The model under review builds one solid part; all positions refer to its coordinate system, in mm. Face numbers are marked on the shaded views. Coordinates: 2 decimals unless noted, no trailing zeros. Loops run counter-clockwise (first coordinate to the right, second up) from the corner with the lowest first, then second, coordinate; pieces in that order, holes last. Notation, with made-up numbers: M 65,-35 L 113,-35 A26 cw 113,-10 Z; hole C 10.5,32 d8. An arc over 180 degrees is marked long. Use CSV: the item, a comma, the result in double quotes. Start each with the question number.
from build123d import *

# Parameters (mm, degrees)
SKETCH1_R           = 4
SKETCH1_R_2         = 2.45
BOSS_EXTRUDE1_DEPTH = 8
SKETCH2_R           = 6
BOSS_EXTRUDE2_DEPTH = 2
FILLET1_R           = 1
CUT_EXTRUDE1_REACH  = 15.115
SKETCH3_R           = 2.45
CHAMFER1_SIZE       = 1


with BuildPart() as part:
    # Sketch1 → Boss-Extrude1 (new body)
    with BuildSketch(Plane(origin=(0, 0, 0), x_dir=(1, 0, 0), z_dir=(0, 1, 0))):
        with Locations(Location((0, 0, 0), (0, 0, 270))):
            Circle(SKETCH1_R)
        with Locations(Location((0, 0, 0), (0, 0, 270))):
            Circle(SKETCH1_R_2, mode=Mode.SUBTRACT)
    extrude(amount=BOSS_EXTRUDE1_DEPTH)

    # Sketch2 → Boss-Extrude2 (add)
    with BuildSketch(Plane(origin=(0, 8, 0), x_dir=(1, 0, 0), z_dir=(0, 1, 0))):
        with Locations(Location((0, 0, 0), (0, 0, 270))):
            Circle(SKETCH2_R)
    extrude(amount=BOSS_EXTRUDE2_DEPTH)

    # Fillet1
    fillet1_edges = [part.edges().sort_by_distance(p)[0] for p in [
        (0, 8, -6),
        (0, 10, -6),
    ]]
    fillet(fillet1_edges, radius=FILLET1_R - 0.0001)  # a hair under: the kernel refuses the full size

    # Sketch3 → Cut-Extrude1 (cut, up to next)
    with BuildSketch(Plane(origin=(0, 10, 0), x_dir=(1, 0, 0), z_dir=(0, 1, 0)), mode=Mode.PRIVATE) as cut_extrude1_sk1:
        with Locations(Location((0, 0, 0), (0, 0, 270))):
            Circle(SKETCH3_R)
    cut_extrude1_tool1 = extrude(cut_extrude1_sk1.sketch, amount=-CUT_EXTRUDE1_REACH, mode=Mode.PRIVATE) & part.part
    add(cut_extrude1_tool1.solids().sort_by_distance((0, 10, 0))[0], mode=Mode.SUBTRACT)

    # Chamfer1
    chamfer1_edges = [part.edges().sort_by_distance(p)[0] for p in [
        (0, 0, -2.45),
    ]]
    chamfer(chamfer1_edges, length=CHAMFER1_SIZE)


solid = part.part
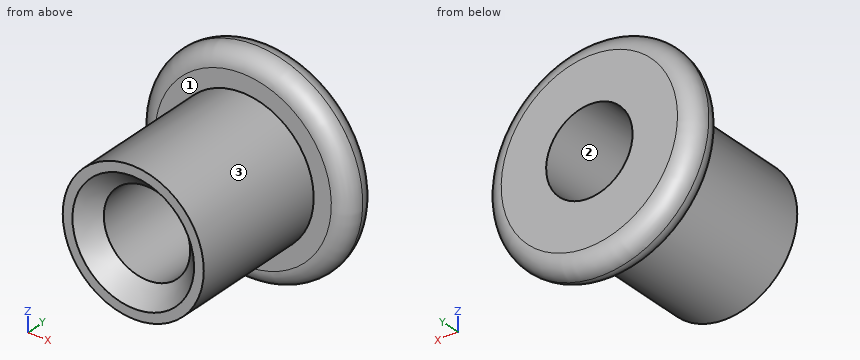
1. To check wall thickness, follow line 1 along X through (y, z) = (5.5, 0); line 2 along X through (y, z) = (8.75, -3.25); line 3 along Z through (x, y) = (-2.25, 1.5). State the ranges of each line that lie inside material, in increasing order.
2. Insertion check: pin 1 Ø4 at (x, y) = (3.5, 5) entering from +Z; pin 2 Ø4 at (x, y) = (3, 4.5) entering from +Z; pin 3 Ø1 at (x, z) = (4.5, 3.5) entering from -Y. Each pin has a flat end and moves straight along its axis. Give the tip position at first contact, or say it passes through.
3. Add section C-C (y = 6.5). Write out the cut boundary in (x, z).
4. Draft analysis for pull direction Z (two halves, no side actions). For the marked faces 1, 2 and 3, state which applies: released by +Z, released by -Z, zero draft, split by the parting line, or undercut.
Solved:
1,line 1,"x = -4 to -2.45, 2.45 to 4"
1,line 2,"x = -5.01 to 5.01"
1,line 3,"z = -3.31 to -0.97, 0.97 to 3.31"
2,pin 1,"stops at z = 3.71"
2,pin 2,"stops at z = 3.87"
2,pin 3,"stops at y = 8.02"
3,outline,"C 0,0 d8; hole C 0,0 d4.9"
4,face 1,"zero draft"
4,face 2,"undercut"
4,face 3,"split by the parting line"
